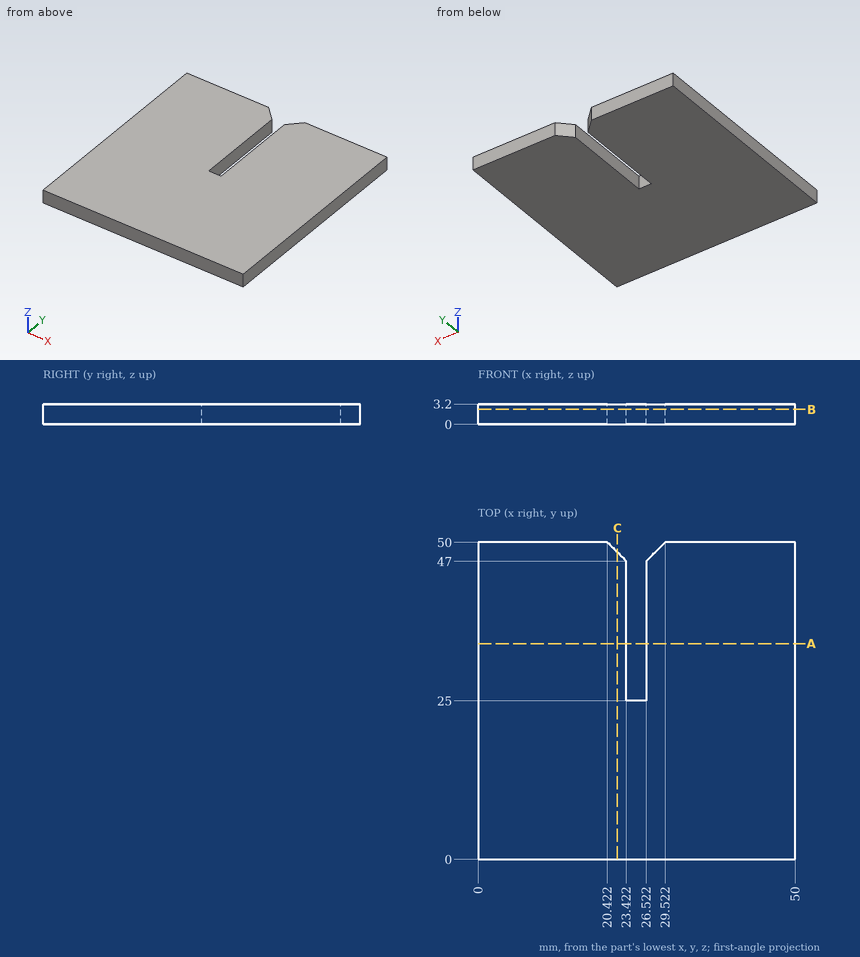
Check sheet for the drawn part. Datum: minimum x, y, z corner. Units: mm. Give positions to 0.01 mm unless a question says otherwise; leave off trailing zeros. Loops run counter-clockwise (first coordinate to the right, second up) from the corner with the lowest first, then second, coordinate; pieces in that order, holes last.
1) Sectioned sample at A-A, the plane y = 34. Enter the section's corners in (x, z), then the cut area to 3 significant figures.
2) Thickness scan on line 1 along X through (y, z) = (41.5, 2.15); line 2 along Y through (x, z) = (27, 2.65). Record the ranges inside material, lowest first.
3) Sectioned sample at B-B, the plane z = 2.35. Enter the section's corners in (x, y).
4) Sectioned sample at C-C, the plane x = 22. Enter the section's corners in (y, z).
5) Depth check by flat-ended pin: pin 1 Ø6 at (x, y) = (20.5, 29.5) entering from -Z; pin 2 Ø1.5 at (x, z) = (25.5, 1) entering from +Y. Enter the tip coordinate at first touch or a pass-through.
Answers:
1. outline: (0, 0) - (23.42, 0) - (23.42, 3.2) - (0, 3.2) - close; (26.52, 0) - (50, 0) - (50, 3.2) - (26.52, 3.2) - close
1. area: 150 mm2
2. line 1: x = 0 to 23.42, 26.52 to 50
2. line 2: y = 0 to 47.48
3. outline: (0, 0) - (50, 0) - (50, 50) - (29.52, 50) - (26.52, 47) - (26.52, 25) - (23.42, 25) - (23.42, 47) - (20.42, 50) - (0, 50) - close
4. outline: (0, 0) - (48.42, 0) - (48.42, 3.2) - (0, 3.2) - close
5. pin 1: stops at z = 0
5. pin 2: stops at y = 25
